The listing builds one solid part. Answer for the finished solid, in the listing's coordinates (mm). Face numbers are marked on the shaded views. A direction names the side the tool comes from. Round coordinates to 2 decimals unless told otherwise and drop trailing zeros. Write each loop counter-clockwise with the first axis right and the second up, starting at its lowest first coordinate (ties: lowest second). Pieces come first, ordered by that corner, then holes.
(1) Find the intervals of material crossed by probe 1 along X at (y, z) = (22.5, -15.5); probe 2 along X at (y, z) = (77.5, -18); probe 3 along Y at (x, z) = (-8.5, -26.5), in increasing order.
(2) Each of these flat-tipped pins is pushed along its axis until it touches: pin 1 Ø6 at (y, z) = (87, 8) entering from +X; pin 2 Ø0.8 at (x, z) = (109, 4.5) entering from +Y; pin 3 Ø1 at (x, z) = (-62.5, 12.5) entering from +Y. Where does it stop, or does it pass through?
(3) A cutting plane is placed at A-A, the plane y = 15.5. Give the vertices of the cut face in (x, z), and give its area (3 significant figures).
(4) The mould has two halves that part along X. Classify the marked faces 3, 4 and 5: +X half, -X half, draft (parallel to the pull), parting line (faces both ways), or undercut.
(5) A cutting plane is placed at D-D, the plane y = 52. Give the vertices of the cut face in (x, z), and give its area (3 significant figures).
(6) A cutting plane is placed at C-C, the plane x = 33. Give the vertices of the cut face in (y, z), and give its area (3 significant figures).
(7) For the marked faces 1 and 2, determine the directions among +Z, -Z, +X, -X, +Y, -Y from which every point of the face is accessible in a straight line to the end or side of a thin tool.
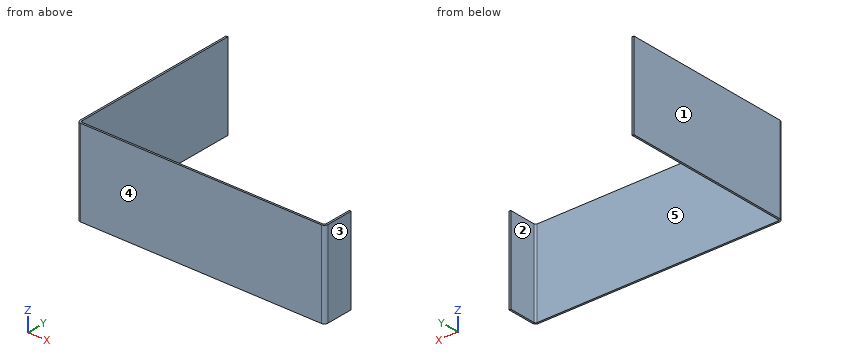
from build123d import *

# Parameters (mm, degrees)
SKETCH1_W                    = 215.9
SKETCH1_H                    = 76.2
BASE_FLANGE1_DEPTH           = 1.5875
EDGE_FLANGE1_STRIP_W         = 9.525
EDGE_FLANGE1_STRIP_H         = 1.5875
EDGE_FLANGE1_STRIP_CUT_DEPTH = 76.2
EDGE_FLANGE1_DEPTH           = 76.2
EDGE_FLANGE3_STRIP_W         = 9.525
EDGE_FLANGE3_STRIP_H         = 1.5875
EDGE_FLANGE3_STRIP_CUT_DEPTH = 76.2
EDGE_FLANGE3_DEPTH           = 76.2


# Sheet-metal steps are written as plain solids
with BuildPart() as part:
    # Sketch1 → Base-Flange1 (new body)
    with BuildSketch(Plane(origin=(0, 0, 0), x_dir=(1, 0, 0), z_dir=(0, 1, 0))):
        Rectangle(SKETCH1_W, SKETCH1_H)
    extrude(amount=-BASE_FLANGE1_DEPTH)

    # Edge-Flange1 strip (across the edge) → Edge-Flange1 strip cut (cut)
    with BuildSketch(Plane(origin=(-107.95, 0, -38.1), x_dir=(1, 0, 0), z_dir=(0, 0, 1))):
        with Locations((-3.175, -0.79375)):
            Rectangle(EDGE_FLANGE1_STRIP_W, EDGE_FLANGE1_STRIP_H)
    extrude(amount=EDGE_FLANGE1_STRIP_CUT_DEPTH, mode=Mode.SUBTRACT)

    # Edge-Flange1 section (across the edge) → Edge-Flange1 (add)
    with BuildSketch(Plane(origin=(-107.95, 0, -38.1), x_dir=(1, 0, 0), z_dir=(0, 0, 1))):
        with BuildLine():
            Line((-1.5875, 1.5875), (-1.5875, 152.4))
            Line((-1.5875, 152.4), (0, 152.4))
            Line((0, 152.4), (0, 1.5875))
            ThreePointArc((0, 1.5875), (0.464967985, 0.464967985), (1.5875, 0))
            Line((1.5875, 0), (1.5875, -1.5875))
            ThreePointArc((1.5875, -1.5875), (-0.65756403, -0.65756403), (-1.5875, 1.5875))
        make_face()
    extrude(amount=EDGE_FLANGE1_DEPTH)

    # Edge-Flange3 strip (across the edge) → Edge-Flange3 strip cut (cut)
    with BuildSketch(Plane(origin=(107.95, 0, 38.1), x_dir=(-1, 0, 0), z_dir=(0, 0, -1))):
        with Locations((-3.175, -0.79375)):
            Rectangle(EDGE_FLANGE3_STRIP_W, EDGE_FLANGE3_STRIP_H)
    extrude(amount=EDGE_FLANGE3_STRIP_CUT_DEPTH, mode=Mode.SUBTRACT)

    # Edge-Flange3 section (across the edge) → Edge-Flange3 (add)
    with BuildSketch(Plane(origin=(107.95, 0, 38.1), x_dir=(-1, 0, 0), z_dir=(0, 0, -1))):
        with BuildLine():
            Line((-1.5875, 1.5875), (-1.5875, 25.4))
            Line((-1.5875, 25.4), (0, 25.4))
            Line((0, 25.4), (0, 1.5875))
            ThreePointArc((0, 1.5875), (0.464967985, 0.464967985), (1.5875, 0))
            Line((1.5875, 0), (1.5875, -1.5875))
            ThreePointArc((1.5875, -1.5875), (-0.65756403, -0.65756403), (-1.5875, 1.5875))
        make_face()
    extrude(amount=EDGE_FLANGE3_DEPTH)


solid = part.part
Solutions:
1. probe 1: x = -109.54 to -107.95, 107.95 to 109.54
1. probe 2: x = -109.54 to -107.95
1. probe 3: y = -1.59 to 0
2. pin 1: stops at x = -107.95
2. pin 2: stops at y = 25.4
2. pin 3: stops at y = 0
3. outline: (-109.54, -38.1) - (-107.95, -38.1) - (-107.95, 38.1) - (-109.54, 38.1) - close; (107.95, -38.1) - (109.54, -38.1) - (109.54, 38.1) - (107.95, 38.1) - close
3. area: 242 mm2
4. face 3: +X half
4. face 4: draft
4. face 5: undercut
5. outline: (-109.54, -38.1) - (-107.95, -38.1) - (-107.95, 38.1) - (-109.54, 38.1) - close
5. area: 121 mm2
6. outline: (-1.59, -38.1) - (0, -38.1) - (0, 38.1) - (-1.59, 38.1) - close
6. area: 121 mm2
7. face 1: +Z, -Z, -X, +Y, -Y
7. face 2: +Z, -Z, +Y
